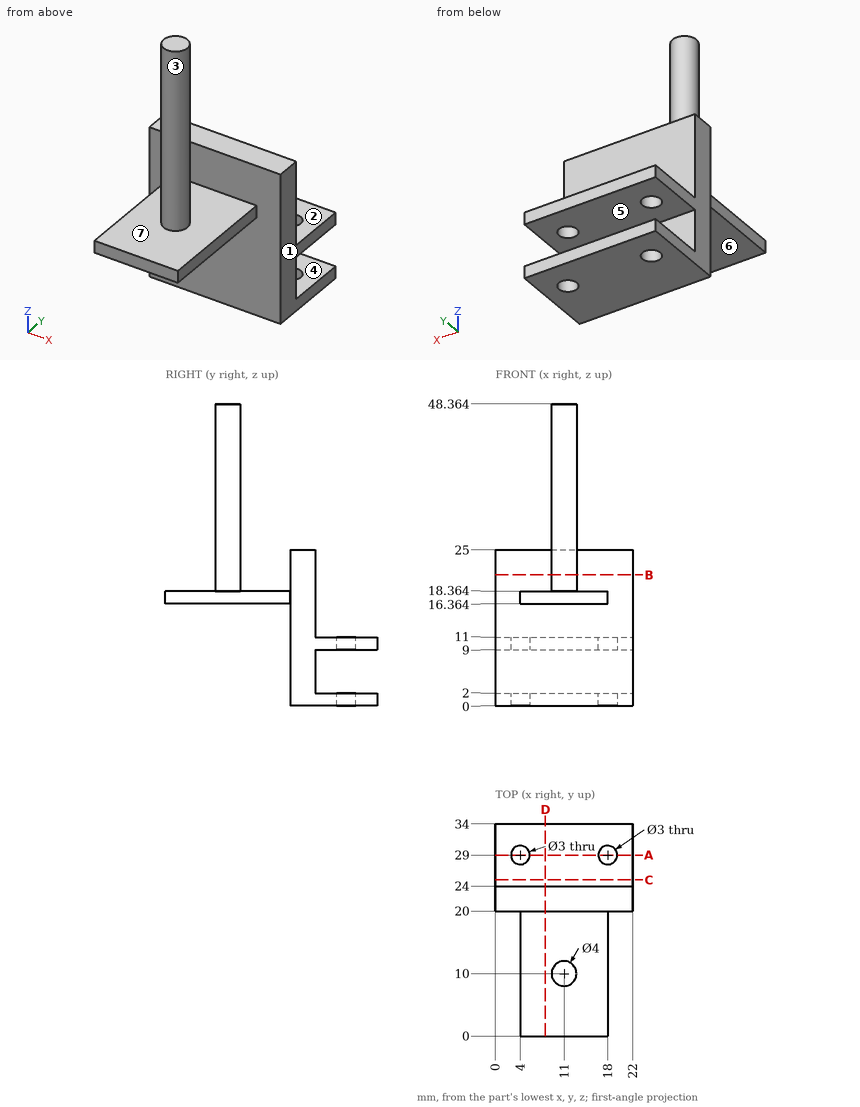
Can you work these out from the drawing? Everything is in mm from the part's minimum corner. A direction names the side the tool comes from. Give positions to 0.01 mm unless a question says otherwise; leave off trailing zeros. Order: outer loops, then holes, each group sorted by start corner. A loop starts at its lowest first (then second) coordinate and runs counter-clockwise, first axis right, second up. Notation, with made-up numbers: M 74.5,-8.75 L 78.5,-8.75 A17 cw 78.5,5.25 Z; hole C -37.5,82.25 d9. An arc over 180 degrees is marked long. Use a Markdown table: item, result. Add a question column.
Item 1: For the marked faces 1, 2, 3 and 4, which set-ups out of +Z, -Z, +X, -X, +Y, -Y let a thin tool reach every point of the face, with its end or its side?
Item 2: We'd pull the mould along Z, two halves only. Please class the marked faces 5, 6 and 7: +Z half, -Z half, draft (parallel to the pull), parting line (faces both ways), or undercut.
Item 3: If I drill on L1, parallel to Z at x = 8.5, y = 27.5; L2, parallel to Y at x = 18, z = 0.4; L3, parallel to Y at x = 15, z = 18.5, over which ranges is the centre line in solid material (lowest first)? Write a range as [from, to].
Item 4: Suppose I cut it at D-D (x = 8). List the corners of the cut face in (y, z) for me.
Item 5: Suppose I cut it at A-A (y = 29). List the corners of the cut face in (x, z) for me.
Item 6: Will these pins go through, and if not, where does the flat tip stop? pin 1 (8 mm diameter, centred on x = 7, y = 31, fed in from +Z); pin 2 (3 mm diameter, centred on x = 7, y = 22.5, fed in from +Z); pin 3 (5 mm diameter, centred on x = 19, z = 21.5, fed in from -Y); pin 4 (8 mm diameter, centred on x = 2.5, z = 41, fed in from -Y).
Item 7: Suppose I cut it at B-B (z = 21). List the corners of the cut face in (x, y) for me, then the cut area to 3 significant figures.
Item 8: Suppose I cut it at C-C (y = 25). List the corners of the cut face in (x, z) for me.
Answer sheet:
| question | item | result |
|---|---|---|
| 1 | face 1 | +Z, -Z, +X, +Y, -Y |
| 1 | face 2 | +Z, +X, -X, +Y |
| 1 | face 3 | +Z |
| 1 | face 4 | +X, -X, +Y |
| 2 | face 5 | undercut |
| 2 | face 6 | -Z half |
| 2 | face 7 | +Z half |
| 3 | L1 | z = [0, 2], [9, 11] |
| 3 | L2 | y = [20, 27.5], [30.5, 34] |
| 3 | L3 | y = [20, 24] |
| 4 | outline | M 0,16.36 L 20,16.36 L 20,0 L 34,0 L 34,2 L 24,2 L 24,9 L 34,9 L 34,11 L 24,11 L 24,25 L 20,25 L 20,18.36 L 0,18.36 Z |
| 5 | outline | M 0,0 L 2.5,0 L 2.5,2 L 0,2 Z; M 0,9 L 2.5,9 L 2.5,11 L 0,11 Z; M 5.5,0 L 16.5,0 L 16.5,2 L 5.5,2 Z; M 5.5,9 L 16.5,9 L 16.5,11 L 5.5,11 Z; M 19.5,0 L 22,0 L 22,2 L 19.5,2 Z; M 19.5,9 L 22,9 L 22,11 L 19.5,11 Z |
| 6 | pin 1 | stops at z = 11 |
| 6 | pin 2 | stops at z = 25 |
| 6 | pin 3 | stops at y = 20 |
| 6 | pin 4 | passes through |
| 7 | outline | M 0,20 L 22,20 L 22,24 L 0,24 Z; C 11,10 d4 |
| 7 | area | 101 mm² |
| 8 | outline | M 0,0 L 22,0 L 22,2 L 0,2 Z; M 0,9 L 22,9 L 22,11 L 0,11 Z |
